```python
from build123d import *

# Parameters (mm, degrees)
SKETCH1_6_R         = 25
BOSS_EXTRUDE3_DEPTH = 5


with BuildPart() as part:
    # Sketch1<6> → Boss-Extrude3 (new, symmetric)
    with BuildSketch(Plane.XY):
        with BuildLine():
            Line((0, 125), (41, 53.98591689))
            ThreePointArc((41, 53.98591689), (29.653041557, 11.639425428), (71.999407886, 0.292000007))
            ThreePointArc((71.999407886, 0.292000007), (60.81182851, -38.5476525), (30.460070741, -65.23943662))
            ThreePointArc((30.460070741, -65.23943662), (0, -40), (-30.460070741, -65.23943662))
            ThreePointArc((-30.460070741, -65.23943662), (-60.81182851, -38.5476525), (-71.999407886, 0.292000007))
            ThreePointArc((-71.999407886, 0.292000007), (-29.653041557, 11.639425428), (-41, 53.98591689))
            Line((-41, 53.98591689), (0, 125))
        make_face()
        Circle(SKETCH1_6_R, mode=Mode.SUBTRACT)
    extrude(amount=BOSS_EXTRUDE3_DEPTH, both=True)


solid = part.part
```
Read the model definition and answer for the solid it produces. Units are mm, in the model's axes. Coordinates: 2 decimals unless noted, no trailing zeros. Order: outer loops, then holes, each group sorted by start corner. A loop starts at its lowest first (then second) coordinate and runs counter-clockwise, first axis right, second up. Notation, with made-up numbers: (26.5, -11) - (82.5, -11) arc R24 ccw to (82.5, 17) - close; hole circle Ø7 at (-29.5, -18.75). An arc over 180 degrees is marked (long way). Answer as a JSON object with one key per item and string values. Group by question number.
Item 1: Section C-C (x = 37) is taken. Give the vertices of the cut face in (y, z).
Item 2: The mould has two halves that part along Y. Classify faces 1 (the face through (1, 31, -5)), 2 (the face through (-20.787, 88.996, 0.07)), 3 (the face through (29.32, 12.23, 0.07)): +Y half, -Y half, draft (parallel to the pull), parting line (faces both ways), or undercut.
Item 3: Section B-B (y = 16.5) is taken. Give the vertices of the cut face in (x, z).
Item 4: Section D-D (y = -33) is taken. Give the vertices of the cut face in (x, z).
Item 5: Flat-ended cylindrical pins translate along their axes: P1, Ø1, axis at y = 57, z = 3.5, coming from the -X side; P2, Ø6, axis at x = -11.5, z = -2, coming from the +Y side; P3, Ø3, axis at x = 24.5, z = 3, coming from the +Y side. Find the tip coordinate at first contact, or state that the pin passes through.
Item 6: Section A-A (z = 0.75) is taken. Give the vertices of the cut face in (x, y), plus the area to 3 significant figures.
Item 7: Consider probe 1 along Y at (x, z) = (0, 2); probe 2 along Y at (x, z) = (-8.5, 2); probe 3 along X at (y, z) = (26, -3.5). Determine where each line is inside the solid, lowest interval first. Write a range as from..to.
Results are:
{
 "1": {"outline": "(-61.77, -5) - (3.04, -5) - (3.04, 5) - (-61.77, 5) - close; (51.24, -5) - (60.91, -5) - (60.91, 5) - (51.24, 5) - close"},
 "2": {"face 1": "draft", "face 2": "+Y half", "face 3": "undercut"},
 "3": {"outline": "(-27.38, -5) - (-18.78, -5) - (-18.78, 5) - (-27.38, 5) - close; (18.78, -5) - (27.38, -5) - (27.38, 5) - (18.78, 5) - close"},
 "4": {"outline": "(-63.99, -5) - (63.99, -5) - (63.99, 5) - (-63.99, 5) - close"},
 "5": {"P1": "stops at x = -39.55", "P2": "stops at y = 110.28", "P3": "stops at y = 85.16"},
 "6": {"outline": "(-72, 0.29) arc R72 ccw to (-30.46, -65.24) arc R31 cw to (30.46, -65.24) arc R72 ccw to (72, 0.29) arc R31 cw to (41, 53.99) - (0, 125) - (-41, 53.99) arc R31 cw to start; hole circle Ø50 at (0, 0)", "area": "10,700 mm^2"},
 "7": {"probe 1": "y = -40..-25, 25..125", "probe 2": "y = -41.19..-23.51, 23.51..110.28", "probe 3": "x = -25.52..25.52"}
}
